Autodesk Fusion 360 part; units mm, degrees
sketch "Sketch1" plane through (0, 0, 0) normal (0, 0, 1) x (1, 0, 0)
  line L0 (-1.25, 0.25) -> (-0.75, 0.25)
  line L1 (-0.75, 0.25) -> (-0.75, -0.25)
  line L2 (-0.75, -0.25) -> (-1.25, -0.25)
  line L3 (-1.25, -0.25) -> (-1.25, 0.25)
  line L4 (0.75, 0.25) -> (1.25, 0.25)
  line L5 (1.25, 0.25) -> (1.25, -0.25)
  line L6 (1.25, -0.25) -> (0.75, -0.25)
  line L7 (0.75, -0.25) -> (0.75, 0.25)
  dimension "d1" = 0.5
  dimension "d2" = 0.5
  dimension "d3" = 0.5
  dimension "d4" = 0.5
  dimension "d5" = 0.75
  dimension "d6" = 0.75
  dimension "d7" = 0.25
  dimension "d8" = 0.25
extrude "Extrude1" add sketch "Sketch1" against normal blind 3.4 makes body 1 at (1.25, 0.0833, -1.1333) makes body 2 at (-1.0833, 0.25, -1.1333)
sketch "Sketch2" plane through (0, 0, 0) normal (0, 0, 1) x (1, 0, 0)
  line L0 (-2.95, 2.8) -> (2.95, 2.8)
  line L1 (2.95, 2.8) -> (2.95, -1.7)
  line L2 (2.95, -1.7) -> (-2.95, -1.7)
  line L3 (-2.95, -1.7) -> (-2.95, 2.8)
  dimension "d11" = 4.5
  dimension "d12" = 1.7
  dimension "d13" = 5.9
  dimension "d14" = 2.95
extrude "Extrude2" add sketch "Sketch2" along normal blind 1 bodies 1 2
sketch "Sketch3" plane through (0, 0, 1) normal (0, 0, 1) x (-1, 0, 0)
  line L0 (2.95, 1.7) -> (-2.95, 1.7)
  line L1 (-2.95, 1.7) -> (-2.95, -2.8)
  line L2 (-2.95, -2.8) -> (2.95, -2.8)
  line L3 (2.95, -2.8) -> (2.95, 1.7)
  line L4 (2.55, 1.3) -> (-2.55, 1.3)
  line L5 (-2.55, 1.3) -> (-2.55, -2.4)
  line L6 (-2.55, -2.4) -> (2.55, -2.4)
  line L7 (2.55, -2.4) -> (2.55, 1.3)
  dimension "d17" = -0.4
extrude "Extrude3" add sketch "Sketch3" along normal blind 5 bodies 1
sketch "Sketch4" plane through (2.95, 0, 0) normal (1, 0, 0) x (0, 1, 0)
  line L0 (-1.7, 0) -> (2.8, 0)
  line L1 (2.8, 0) -> (2.8, 6)
  line L2 (2.8, 6) -> (-1.7, 6)
  line L3 (-1.7, 6) -> (-1.7, 0)
  line L4 (-0.2, 6) -> (-0.2, 4)
  line L5 (0.8, 6) -> (0.8, 4)
  arc A0 (-0.2, 4) -> (0.8, 4) centre (0.3, 4) ccw
  line L6 (-0.2, 6) -> (0.8, 6)
  dimension "d20" = 2
  dimension "d21" = 1.5
  dimension "d22" = 1
  dimension "d23" = 1
  dimension "d24" = 2
extrude "Extrude4" cut sketch "Sketch4" against normal blind 6 contours L2 L4 L5 A0 L6 bodies 1
sketch "Sketch5" plane through (0, -1.7, 0) normal (0, -1, 0) x (1, 0, 0)
  line L0 (-2.95, 0) -> (2.95, 0)
  line L1 (2.95, 0) -> (2.95, 6)
  line L2 (2.95, 6) -> (-2.95, 6)
  line L3 (-2.95, 6) -> (-2.95, 0)
  line L4 (-2.95, 0.9) -> (2.95, 0.9)
  line L5 (2.95, 0.9) -> (2.95, 0.5)
  line L6 (2.95, 0.5) -> (-2.95, 0.5)
  line L7 (-2.95, 0.5) -> (-2.95, 0.9)
  line L8 (-2.2, 4) -> (-1.2, 4)
  line L9 (-1.2, 4) -> (-1.2, 2)
  line L10 (-1.2, 2) -> (-2.2, 2)
  line L11 (-2.2, 2) -> (-2.2, 4)
  line L12 (1.2, 4) -> (2.2, 4)
  line L13 (2.2, 4) -> (2.2, 2)
  line L14 (2.2, 2) -> (1.2, 2)
  line L15 (1.2, 2) -> (1.2, 4)
  line L16 (-2.95, 0) -> (2.95, 0)
  dimension "d27" = 0.9
  dimension "d28" = 0.4
  dimension "d29" = 1
  dimension "d30" = 1
  dimension "d31" = 2
  dimension "d32" = 2
  dimension "d33" = 0.75
  dimension "d34" = 0.75
  dimension "d35" = 2
  dimension "d36" = 2
extrude "Extrude5" cut sketch "Sketch5" against normal blind 0.4 contours L1 L3 L4 L5 L6 L7 | L8 L9 L10 L11 | L12 L13 L14 L15 bodies 1
sketch "Sketch6" plane through (0, 0, 1) normal (0, 0, 1) x (-1, 0, 0)
  line L0 (2.55, 1.3) -> (-2.55, 1.3)
  line L1 (-2.55, 1.3) -> (-2.55, -2.4)
  line L2 (-2.55, -2.4) -> (2.55, -2.4)
  line L3 (2.55, -2.4) -> (2.55, 1.3)
  line L4 (0.75, 0.25) -> (1.25, 0.25)
  line L5 (1.25, 0.25) -> (1.25, -0.25)
  line L6 (1.25, -0.25) -> (0.75, -0.25)
  line L7 (0.75, -0.25) -> (0.75, 0.25)
  line L8 (-1.25, 0.25) -> (-0.75, 0.25)
  line L9 (-0.75, 0.25) -> (-0.75, -0.25)
  line L10 (-0.75, -0.25) -> (-1.25, -0.25)
  line L11 (-1.25, -0.25) -> (-1.25, 0.25)
extrude "Extrude6" add sketch "Sketch6" along normal blind 4 contours L4 L5 L6 L7 | L8 L9 L10 L11 bodies 1
chamfer "Chamfer1" distance 0.1 angle 45 16 edges at (1.25, 0, 5) (1, 0.25, 5) (0.75, 0, 5) (1, -0.25, 5) (-0.75, 0, 5) (-1, 0.25, 5) (-1.25, 0, 5) (-1, -0.25, 5) (1.25, 0, -3.4) (1, 0.25, -3.4) (0.75, 0, -3.4) (1, -0.25, -3.4) (-0.75, 0, -3.4) (-1, -0.25, -3.4) (-1.25, 0, -3.4) (-1, 0.25, -3.4) on bodies 1
equation "d14 = ( 5.9 / 2 ) * 1 mm"
Source: CAD feature listing. Evaluate the final solid. Frame: model axes, mm. A direction names the side the tool comes from. Give positions to 0.01 mm unless a question says otherwise; leave off trailing zeros. Loops run counter-clockwise (first coordinate to the right, second up) from the corner with the lowest first, then second, coordinate; pieces in that order, holes last. Notation, with made-up numbers: (-31.5, 89.5) -> (-9.5, 89.5) arc R23 ccw to (-9.5, 107.5) -> close; hole circle Ø5 at (0, 51.5). An arc over 180 degrees is marked (long way). Use a Markdown table: item, result. Add a question column.
1) Section query D-D, the plane z = -1.25. Return the cut outline in (x, y), then the cut area to 3 significant figures.
2) Pull-direction query (X, two-part tool) for faces 1 (the face through (2.95, 1, 3)), 2 (the face through (0, -1.7, 3)), 3 (the face through (0, 2.4, 3)); classes: +X half, -X half, draft (parallel to the pull), parting line (faces both ways), or undercut.
3) First-contact query: pin 1 (0.6 mm diameter, centred on x = 1, z = -2.5, fed in from +Y); pin 2 (1.5 mm diameter, centred on x = 1.5, y = 2, fed in from -Z). Flat tips, straight axial feed; report the tip coordinate or a pass-through.
4) Line query: line 1 along X through (y, z) = (-0.2, 1.5); line 2 along X through (y, z) = (2.3, 2); line 3 along X through (y, z) = (-0.15, -1). Output: solid intervals per line, ascending. Write a range as [from, to].
5) Section query A-A, the plane y = -1.4. Return the cut outline in (x, z), then the cut area to 3 significant figures.
6) Section query B-B, the plane z = 3.25. Return the cut outline in (x, y), then the cut area to 3 significant figures.
7) Reachability of faces 4 (the face through (0, 2.8, 3)), 5 (the face through (-2.55, 1, 3)) from +Z, -Z, +X, -X, +Y, -Y: full face, straight path, thin tool, end or side. Return the list, or none.
8) Section query C-C, the plane x = -1.4. Return the cut outline in (y, z), then the cut area to 3 significant figures.
Numbers:
| question | item | result |
|---|---|---|
| 1 | outline | (-1.25, -0.25) -> (-0.75, -0.25) -> (-0.75, 0.25) -> (-1.25, 0.25) -> close; (0.75, -0.25) -> (1.25, -0.25) -> (1.25, 0.25) -> (0.75, 0.25) -> close |
| 1 | area | 0.500 mm2 |
| 2 | face 1 | +X half |
| 2 | face 2 | draft |
| 2 | face 3 | undercut |
| 3 | pin 1 | stops at y = 0.25 |
| 3 | pin 2 | stops at z = 0 |
| 4 | line 1 | x = [-2.95, -2.55], [-1.25, -0.75], [0.75, 1.25], [2.55, 2.95] |
| 4 | line 2 | x = [-2.95, -2.55], [2.55, 2.95] |
| 4 | line 3 | x = [-1.25, -0.75], [0.75, 1.25] |
| 5 | outline | (-2.95, 0) -> (2.95, 0) -> (2.95, 0.5) -> (-2.95, 0.5) -> close; (-2.95, 0.9) -> (2.95, 0.9) -> (2.95, 6) -> (-2.95, 6) -> close; hole (-2.2, 2) -> (-1.2, 2) -> (-1.2, 4) -> (-2.2, 4) -> close; hole (1.2, 2) -> (2.2, 2) -> (2.2, 4) -> (1.2, 4) -> close |
| 5 | area | 29.0 mm2 |
| 6 | outline | (-2.95, -1.7) -> (-2.2, -1.7) -> (-2.2, -1.3) -> (-2.55, -1.3) -> (-2.55, 2.4) -> (2.55, 2.4) -> (2.55, -1.3) -> (2.2, -1.3) -> (2.2, -1.7) -> (2.95, -1.7) -> (2.95, 2.8) -> (-2.95, 2.8) -> close; (-1.25, -0.25) -> (-0.75, -0.25) -> (-0.75, 0.25) -> (-1.25, 0.25) -> close; (-1.2, -1.7) -> (1.2, -1.7) -> (1.2, -1.3) -> (-1.2, -1.3) -> close; (0.75, -0.25) -> (1.25, -0.25) -> (1.25, 0.25) -> (0.75, 0.25) -> close |
| 6 | area | 7.38 mm2 |
| 7 | face 4 | +Z, -Z, +X, -X, +Y |
| 7 | face 5 | +Z |
| 8 | outline | (-1.7, 0) -> (2.8, 0) -> (2.8, 6) -> (2.4, 6) -> (2.4, 1) -> (-1.3, 1) -> (-1.3, 2) -> (-1.7, 2) -> (-1.7, 0.9) -> (-1.3, 0.9) -> (-1.3, 0.5) -> (-1.7, 0.5) -> close; (-1.7, 4) -> (-1.3, 4) -> (-1.3, 6) -> (-1.7, 6) -> close |
| 8 | area | 7.54 mm2 |
